Autodesk Inventor part; units mm, degrees
ref_plane "YZ Plane" through (0, 0, 0) normal (1, 0, 0) x (0, 1, 0)
ref_plane "XZ Plane" through (0, 0, 0) normal (0, 1, 0) x (-1, 0, 0)
ref_plane "XY Plane" through (0, 0, 0) normal (0, 0, 1) x (1, 0, 0)
sketch "Sketch1" plane through (0, 0, 0) normal (0, 0, 1) x (1, 0, 0)
  line L0 (7.5, 3.8038) -> (3.6225, 3.8038)
  arc A0 (1.9153, 4.762) -> (3.6225, 3.8038) centre (3.6225, 5.8038) ccw
  line L1 (1.9153, 4.762) -> (-2.2072, 11.517)
  arc A1 (-2.5, 12.5588) -> (-2.2072, 11.517) centre (-0.5, 12.5588) ccw
  line L2 (-2.5, 12.5588) -> (-2.5, 21.8038)
  arc A2 (-0.5, 23.8038) -> (-2.5, 21.8038) centre (-0.5, 21.8038) ccw
  line L3 (-0.5, 23.8038) -> (7.5, 23.8038)
  line L4 (7.5, 23.8038) -> (7.5, 3.8038)
  spline S0 degree 3 poles (-6.0485, -11.2843) (-6.0213, -11.0209) (-5.9428, -10.7653) (-5.6929, -10.2997) (-5.524, -10.094) (-5.1467, -9.7842) (-4.9505, -9.6718) (-4.5292, -9.5173) (-4.3073, -9.4763) (-4.0832, -9.4731) knots 0 0 0 0 0.079442 0.079442 0.158531 0.158531 0.225919 0.225919 0.293184 0.293184 0.293184 0.293184
  line L5 (-6.0485, -11.2843) -> (-6.563, -16.2598)
  line L6 (-6.563, -16.2598) -> (-6.8849, -19.6266)
  arc A3 (-6.8849, -19.6266) -> (-5.7884, -21.6058) centre (-4.894, -19.817) ccw
  line L7 (17.5, -33.2499) -> (-5.7884, -21.6058)
  line L8 (17.5, 31.9794) -> (17.5, -33.2499)
  arc A4 (4.376, 33.2499) -> (17.5, 31.9794) centre (12.5, 48.7499) ccw
  arc A5 (-1.8324, 56.2463) -> (4.376, 33.2499) centre (12.5, 47.7794) ccw
  line L9 (-1.8324, 56.2463) -> (-17.5, 52.7794)
  line L10 (-17.5, 52.7794) -> (-17.5, 3.0185)
  ellipse E0 centre (-15.5, 3.0185) end of major axis (-15.5, 1.0011) minor radius 2 (-17.5, 3.0185) -> (-15.6888, 1.0101) ccw
  line L11 (-15.6888, 1.0101) -> (-3.1949, -0.1848)
  line L12 (-3.1949, -0.1848) -> (-4.0832, -9.4731)
  circle A6 centre (-12, 26.728) radius 1.25
  circle A7 centre (5.3255, 26.728) radius 1.25
  line L13 (-14, 9.2999) -> (-10, 9.2999)
  line L14 (-14, 15.6999) -> (-14, 9.2999)
  line L15 (-10, 15.6999) -> (-14, 15.6999)
  line L16 (-10, 9.2999) -> (-10, 15.6999)
  line L17 (13.7851, 6.0601) -> (9.7851, 6.0601)
  line L18 (13.7851, -0.3399) -> (13.7851, 6.0601)
  line L19 (9.7851, -0.3399) -> (13.7851, -0.3399)
  line L20 (9.7851, 6.0601) -> (9.7851, -0.3399)
  circle A8 centre (7.1425, -8.6154) radius 1.25
  line L21 (17.5, -33.2499) -> (-17.5, -15.7501)
  line L22 (-17.5, -15.7501) -> (-17.5, -17.9862)
  line L23 (-17.5, -17.9862) -> (17.5, -35.486)
  line L24 (17.5, -35.486) -> (17.5, -33.2499)
  line L25 (-1.4649, 56.8397) -> (-18, 53.1809)
  line L26 (-18, 53.1809) -> (-18, -17.9862)
  line L27 (-18, -17.9862) -> (-17.5, -17.9862)
  line L28 (-17.5, -17.9862) -> (-17.5, 52.7794)
  line L29 (-17.5, 52.7794) -> (-1.8324, 56.2463)
  arc A9 (-1.4649, 56.8397) -> (-1.8324, 56.2463) centre (12.5, 47.7794) ccw
  line L30 (19.5, -37.0206) -> (19.5, 31.9794)
  line L31 (19.5, 31.9794) -> (17.5, 31.9794)
  line L32 (17.5, -37.0206) -> (17.5, 31.9794)
  line L33 (19.5, -37.0206) -> (17.5, -37.0206)
  circle A10 centre (12.5, 47.7794) radius 15.02
  line L34 (-1.4649, 56.8397) -> (-11.9805, 54.5129)
  line L35 (-11.9805, 54.5129) -> (26.5324, 63.5095)
  line L36 (17.5, 31.9794) -> (17.5, 20.7849)
  line L37 (17.5, 20.7849) -> (17.5, 78.444)
  circle A11 centre (12.5, 47.7794) radius 12.1257
  line L38 (-17.5, -15.7501) -> (-17.5, 52.7794)
  line L39 (-1.8324, 56.2463) -> (11.2654, 59.1445)
  line L40 (11.2654, 59.1445) -> (26.5324, 62.5227)
  circle A12 centre (12.5, 47.7794) radius 11.3634
  point P0 (0, 0)
  point P1 (17.5, 57.9837)
  point P2 (10.0449, 58.8745)
extrude "Extrusion1" add sketch "Sketch1" along normal blind 0.5 contours L0 A0 L1 A1 L2 A2 L3 L4 | L5 L6 A3 L21 L28 E0 L11 L12 S0 | S0 L12 L11 E0 L10 L9 A5 A4 L8 L7 A3 L6 L5 | L39 A10 L37 A4 A5 | L39 A11 L37 A10 | L39 A12 L37 A11 | A12 L37 | L14 L15 L16 L13 | L18 L19 L20 L17 picked at (9.8401, 51.5561)
sketch "Sketch2" plane through (0, 0, 0.5) normal (0, 0, 1) x (1, 0, 0)
  line L0 (17.5, -33.2499) -> (17.5, 57.9837)
  arc A0 (17.5, 57.9837) -> (10.0449, 58.8745) centre (12.5, 47.7794) ccw
  line L1 (10.0449, 58.8745) -> (-17.5, 52.7794)
  line L2 (-17.5, 52.7794) -> (-17.5, -15.7501)
  line L3 (-17.5, -15.7501) -> (17.5, -33.2499)
  circle A1 centre (-12, 26.728) radius 1.25
  circle A2 centre (5.3255, 26.728) radius 1.25
  circle A3 centre (7.1425, -8.6154) radius 1.25
  point P0 (0, 0)
extrude "Extrusion2" add sketch "Sketch2" against normal blind 0.5 contours A1 | A2 | A3
properties part number "pokrywa lewa" material "Stal miękka, spawana"
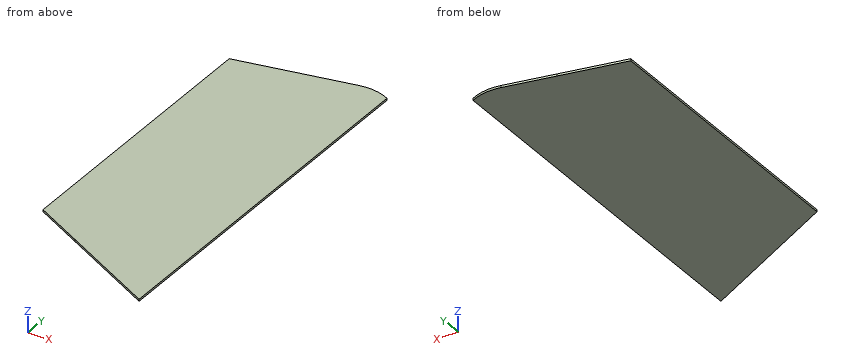
Check sheet for the modelled part. Datum: model origin and axes. Units: mm. Coordinates: 2 decimals unless noted, no trailing zeros. Loops run counter-clockwise (first coordinate to the right, second up) from the corner with the lowest first, then second, coordinate; pieces in that order, holes last.
1) Sectioned sample at B-B (x = -10.5). Record the boundary of the cut face in (y, z), and give its area (3 significant figures).
2) Material ranges on probe 1 along Y at (x, z) = (-9, 0.45); probe 2 along Y at (x, z) = (-3, 0.45), recorded low to high.
3) Sectioned sample at C-C (y = -18). Record the boundary of the cut face in (x, z).
4) Sectioned sample at A-A (z = 0.2). Record the boundary of the cut face in (x, y), and give its area (3 significant figures).
Check sheet entries:
1. outline: (-19.25, 0) - (54.33, 0) - (54.33, 0.5) - (-19.25, 0.5) - close
1. area: 36.8 mm2
2. probe 1: y = -20 to 54.66
2. probe 2: y = -23 to 55.99
3. outline: (-13, 0) - (17.5, 0) - (17.5, 0.5) - (-13, 0.5) - close
4. outline: (-17.5, -15.75) - (-5.79, -21.61) - (17.5, -33.25) - (17.5, 57.98) arc R11.36 ccw to (10.04, 58.87) - (-1.83, 56.25) - (-17.5, 52.78) - close
4. area: 2,830 mm2
